Could you check a few things on this model? Use its own coordinates, in mm. Face numbers are marked on the shaded views. A direction names the side the tool comes from. Round coordinates to 2 decimals unless told otherwise and drop trailing zeros. Write each loop counter-clockwise with the first axis right and the second up, starting at its lowest first coordinate (ties: lowest second). Pieces come first, ordered by that corner, then holes. Notation, with made-up numbers: M -39,-6 L 8,-6 A24 ccw 8,14 Z; hole C 19,37 d7. An arc over 180 degrees is marked long. One line per item, written item: value. Start each with the question number.
(1) I'm going to push flat-ended pins straight in: pin 1 Ø3.5 at (x, z) = (27.2, 32) entering from +Y; pin 2 Ø1 at (y, z) = (-3.5, 31.5) entering from -X; pin 3 Ø4 at (x, z) = (21.5, 8) entering from -Y; pin 4 Ø4 at (x, z) = (21, 32) entering from +Y. Where does each tip first touch, or does it pass through?
(2) I want a section at A-A on y = -4. Please give me the cut outline in (x, z) (1 decimal).
(3) Which directions (+Z, -Z, +X, -X, +Y, -Y) give clear straight access to the entire face, cutting with the end or side of a thin tool? Please do the marked faces 4, 5, 6, 7 and 8.
(4) If I drill on L1, parallel to Z at x = 47.2, y = 0.9 (3 decimals); L2, parallel to Y at x = 41, z = 9; L3, parallel to X at y = -2, z = 2.5, over which ranges is the centre line in solid material (lowest first)?
(5) I want a section at D-D on x = 0. Please give me the cut outline in (y, z).
(6) Thinking about a two-plate mould opening in Y: for the marked faces 1, 2 and 3, which applies, released by +Y, released by -Y, zero draft, split by the parting line, or undercut?
(7) I want a section at C-C on y = 0. Please give me the cut outline in (x, z) (3 decimals).
(8) I want a section at B-B on z = 32. Please give me the cut outline in (x, y) (3 decimals), and give its area (3 significant figures).
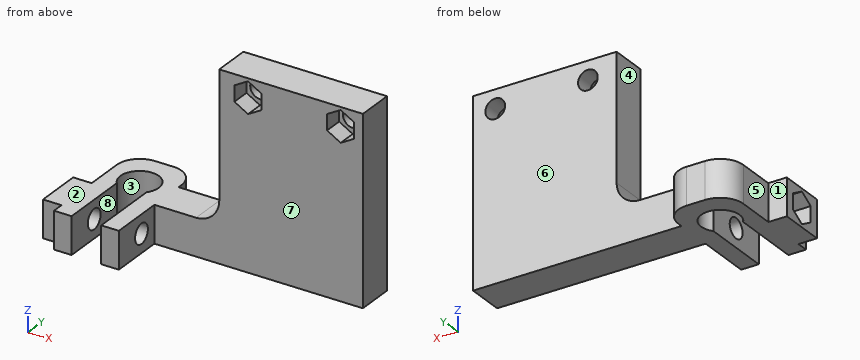
```python
from build123d import *

# Parameters (mm, degrees)
F1_DEPTH  = 4
F2_R      = 5
F3_R      = 2.125
F4_DEPTH  = 25
F5_W      = 10
F5_H      = 8
F6_DEPTH  = 4
F7_W      = 45
F7_H      = 8
F8_DEPTH  = 36
F9_W      = 45
F9_H      = 8
F10_DEPTH = 4
F11_R     = 2.125
F12_DEPTH = 25
F14_DEPTH = 4
F15_W     = 14
F15_H     = 32
F16_DEPTH = 25
F17_R     = 5


with BuildPart() as f1:
    # F0 (on Top) → F1 (new body, symmetric)
    with BuildSketch(Plane.XY):
        with BuildLine():
            ThreePointArc((-3.2, -2.642442), (0, 4.15), (3.2, -2.642442))
            Line((3.2, -2.642442), (3.2, -17.642442))
            Line((3.2, -17.642442), (7, -17.642442))
            Line((7, -17.642442), (7, -2.65))
            Line((7, -2.65), (7, -1.85))
            Line((7, -1.85), (7, 2.35))
            Line((7, 2.35), (7, 8.15))
            Line((7, 8.15), (-7, 8.15))
            Line((-7, 8.15), (-7, 3.15))
            Line((-7, 3.15), (-7, -17.642442))
            Line((-7, -17.642442), (-3.2, -17.642442))
            Line((-3.2, -17.642442), (-3.2, -2.642442))
        make_face()
    extrude(amount=F1_DEPTH, both=True)

    # F2
    f2_edges = [f1.edges().sort_by_distance(p)[0] for p in [
        (-7, 8.15, 0),
    ]]
    fillet(f2_edges, radius=F2_R)

    # F3 (on face) → F4 (cut)
    with BuildSketch(Plane(origin=(-7, 0, 0), x_dir=(0, -1, 0), z_dir=(-1, 0, 0))):
        with Locations((10.142442, 0)):
            Circle(F3_R)
    extrude(amount=-F4_DEPTH, mode=Mode.SUBTRACT)

    # F5 (on face) → F6 (join)
    with BuildSketch(Plane(origin=(-7, 0, 0), x_dir=(0, -1, 0), z_dir=(-1, 0, 0))):
        with Locations((10.142442, 0)):
            Rectangle(F5_W, F5_H)
        Polygon((10.142442, 3.377499), (13.067442, 1.68875), (13.067442, -1.68875), (10.142442, -3.377499), (7.217442, -1.68875), (7.217442, 1.68875), align=None, mode=Mode.SUBTRACT)
    extrude(amount=F6_DEPTH)

    # F7 (on Top) → F8 (join)
    with BuildSketch(Plane.XY):
        with Locations((29.5, -1.85)):
            Rectangle(F7_W, F7_H)
    extrude(amount=F8_DEPTH)

    # F9 (on face) → F10 (join)
    with BuildSketch(Plane(origin=(0, 0, 0), x_dir=(1, 0, 0), z_dir=(0, 0, -1))):
        with Locations((29.5, 1.85)):
            Rectangle(F9_W, F9_H)
    extrude(amount=F10_DEPTH)

    # F11 (on face) → F12 (cut)
    with BuildSketch(Plane.XZ.offset(5.85)):
        with Locations((27.2, 32)):
            Circle(F11_R)
        with Locations((47.2, 32)):
            Circle(F11_R)
    extrude(amount=-F12_DEPTH, mode=Mode.SUBTRACT)

    # F13 (on face) → F14 (cut)
    with BuildSketch(Plane.XZ.offset(5.85)):
        Polygon((30.125, 30.31125), (30.125, 33.68875), (27.2, 35.377499), (24.275, 33.68875), (24.275, 30.31125), (27.2, 28.622501), align=None)
        Polygon((44.275, 33.68875), (44.275, 30.31125), (47.2, 28.622501), (50.125, 30.31125), (50.125, 33.68875), (47.2, 35.377499), align=None)
    extrude(amount=-F14_DEPTH, mode=Mode.SUBTRACT)

    # F15 (on face) → F16 (cut)
    with BuildSketch(Plane(origin=(0, 2.15, 0), x_dir=(-1, 0, 0), z_dir=(0, 1, 0))):
        with Locations((-14, 20)):
            Rectangle(F15_W, F15_H)
    extrude(amount=-F16_DEPTH, mode=Mode.SUBTRACT)

    # F17
    f17_edges = [f1.edges().sort_by_distance(p)[0] for p in [
        (21, -1.85, 4),
        (7, 8.15, 0),
    ]]
    fillet(f17_edges, radius=F17_R)


solid = f1.part
```
Found:
1. pin 1: passes through
1. pin 2: stops at x = 21
1. pin 3: stops at y = -5.85
1. pin 4: stops at y = 2.15
2. outline: M -7,-4 L -3.2,-4 L -3.2,4 L -7,4 Z; M 3.2,-4 L 52,-4 L 52,36 L 21,36 L 21,9 A5 cw 16,4 L 3.2,4 Z; hole M 24.3,30.3 L 27.2,28.6 L 30.1,30.3 L 30.1,33.7 L 27.2,35.4 L 24.3,33.7 Z; hole M 44.3,30.3 L 47.2,28.6 L 50.1,30.3 L 50.1,33.7 L 47.2,35.4 L 44.3,33.7 Z
3. face 4: +Z, -X, +Y, -Y
3. face 5: +Z, -Z, -X, +Y
3. face 6: +Z, -Z, +X, +Y
3. face 7: +Z, -Z, +X, -Y
3. face 8: +Z, -Z, -Y
4. L1: z = -4 to 29.875, 34.125 to 36
4. L2: y = -5.85 to 2.15
4. L3: x = -7 to -3.64, 3.64 to 52
5. outline: M 4.15,-4 L 8.15,-4 L 8.15,4 L 4.15,4 Z
6. face 1: released by +Y
6. face 2: zero draft
6. face 3: undercut
7. outline: M -7,-4 L -4.15,-4 L -4.15,4 L -7,4 Z; M 4.15,-4 L 52,-4 L 52,36 L 21,36 L 21,9 A5 cw 16,4 L 4.15,4 Z; hole C 27.2,32 d4.25; hole C 47.2,32 d4.25
8. outline: M 21,-5.85 L 24.275,-5.85 L 24.275,-1.85 L 25.075,-1.85 L 25.075,2.15 L 21,2.15 Z; M 29.325,-1.85 L 30.125,-1.85 L 30.125,-5.85 L 44.275,-5.85 L 44.275,-1.85 L 45.075,-1.85 L 45.075,2.15 L 29.325,2.15 Z; M 49.325,-1.85 L 50.125,-1.85 L 50.125,-5.85 L 52,-5.85 L 52,2.15 L 49.325,2.15 Z
8. area: 167 mm²
